Design review of the part shown in the three views and the two pictorial views. Dimensions are in mm from the part's minimum x, y and z. A direction names the side the tool comes from. Coordinates: 2 decimals unless noted, no trailing zeros. Loops run counter-clockwise (first coordinate to the right, second up) from the corner with the lowest first, then second, coordinate; pieces in that order, holes last. Notation, with made-up numbers: (-31.75, 77.25) -> (23.25, 77.25) arc R14 ccw to (23.25, 87.25) -> close; hole circle Ø2 at (-24, -22.5). An arc over 180 degrees is marked (long way). Answer in a Markdown table with one row per item.
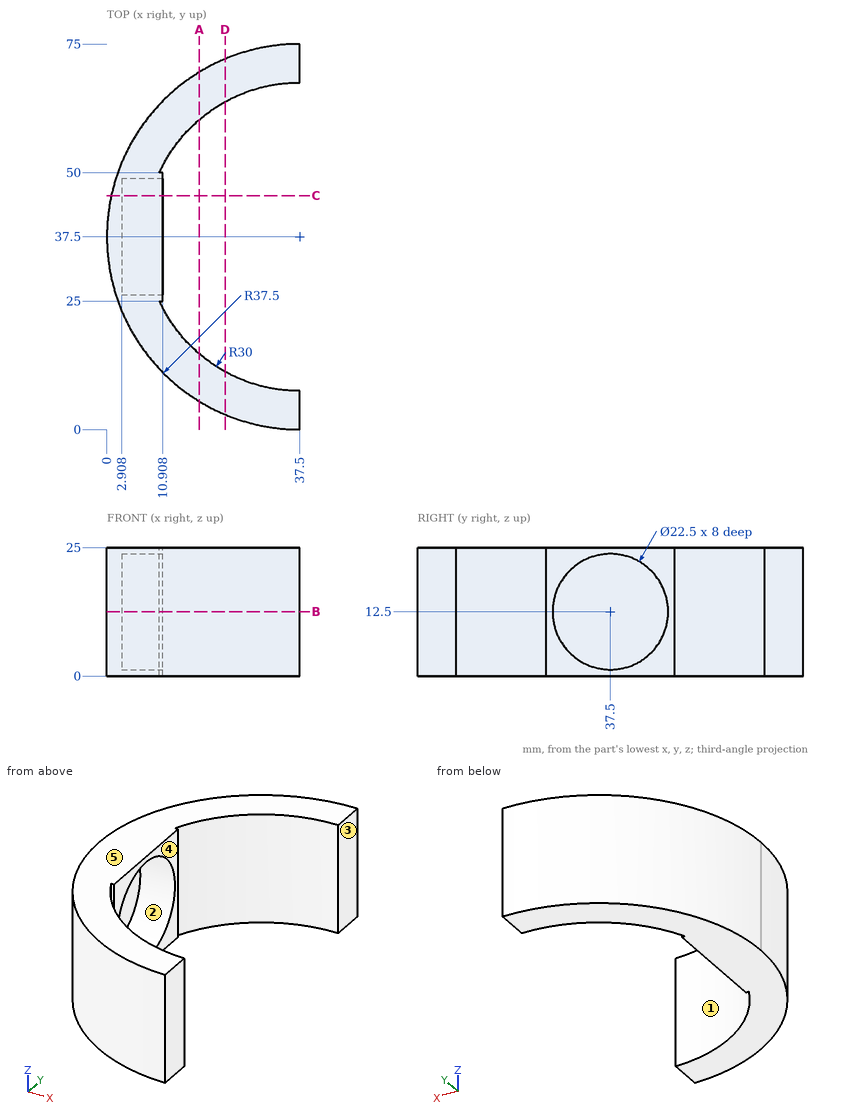
(1) Take a section at B-B on z = 12.5. Give the boundary of the cut face in (x, y), and give its area (3 significant figures).
Evaluation:
| item | result |
|---|---|
| outline | (0, 37.5) arc R37.5 ccw to (37.5, 0) -> (37.5, 7.5) arc R30 cw to (10.23, 25) -> (10.91, 25) -> (10.91, 26.25) -> (2.91, 26.25) -> (2.91, 48.75) -> (10.91, 48.75) -> (10.91, 50) -> (10.23, 50) arc R30 cw to (37.5, 67.5) -> (37.5, 75) arc R37.5 ccw to start |
| area | 678 mm² |
(2) Take a section at C-C on y = 45.5. Give the boundary of the cut face in (x, z), and give its area (3 significant figures).
Evaluation:
| item | result |
|---|---|
| outline | (0.86, 0) -> (10.91, 0) -> (10.91, 4.59) -> (2.91, 4.59) -> (2.91, 20.41) -> (10.91, 20.41) -> (10.91, 25) -> (0.86, 25) -> close |
| area | 125 mm² |
(3) To check wall thickness, follow probe 1 along Z at (x, y) = (6, 37.5); probe 2 along Y at (x, z) = (15.5, 11.25); probe 3 along Y at (x, z) = (17, 16.5). State the ranges of each line that lie inside material, in increasing order.
Evaluation:
| item | result |
|---|---|
| probe 1 | z = 0 to 1.25, 23.75 to 25 |
| probe 2 | y = 7.13 to 17.1, 57.9 to 67.87 |
| probe 3 | y = 6.1 to 15.6, 59.4 to 68.9 |
(4) Draft analysis for pull direction Y (two halves, no side actions). For the marked faces 1, 2 and 3, state which applies: pulls with the +Y half, pulls with the -Y half, needs draft (parallel to the pull), parting line crosses it, or undercut.
Evaluation:
| item | result |
|---|---|
| face 1 | undercut |
| face 2 | undercut |
| face 3 | needs draft |
(5) For pin 1 (0.7 mm diameter, centred on x = 10.5, z = 15, fed in from +Y); pin 2 (12 mm diameter, centred on x = 27, z = 19, fed in from +Y); pin 3 (0.7 mm diameter, centred on x = 10.5, z = 17, fed in from -Y), all flat-tipped, find the tip position at first contact; note any pin that passes through.
Evaluation:
| item | result |
|---|---|
| pin 1 | stops at y = 63.88 |
| pin 2 | stops at y = 74.73 |
| pin 3 | stops at y = 11.12 |
(6) Take a section at D-D on x = 23. Give the boundary of the cut face in (y, z).
Evaluation:
| item | result |
|---|---|
| outline | (2.92, 0) -> (11.24, 0) -> (11.24, 25) -> (2.92, 25) -> close; (63.76, 0) -> (72.08, 0) -> (72.08, 25) -> (63.76, 25) -> close |
(7) Take a section at A-A on x = 18. Give the boundary of the cut face in (y, z).
Evaluation:
| item | result |
|---|---|
| outline | (5.47, 0) -> (14.7, 0) -> (14.7, 25) -> (5.47, 25) -> close; (60.3, 0) -> (69.53, 0) -> (69.53, 25) -> (60.3, 25) -> close |
(8) Tool access review of the marked faces 4 and 5: name each direction out of +Z, -Z, +X, -X, +Y, -Y from which nothing blocks a thin tool from reaching the whole face with its end or side.
Evaluation:
| item | result |
|---|---|
| face 4 | +Z, -Z, +X |
| face 5 | +Z, +X, -X, +Y, -Y |
